```python
from build123d import *

# Parameters (mm, degrees)
ESBO_O1_R                     = 28.25
RESSALTO_EXTRUS_O1_DEPTH      = 12.625
ESBO_O2_R                     = 18.5
CORTE_EXTRUS_O1_DEPTH         = 3.5
ESBO_O3_R                     = 25.75
CORTE_EXTRUS_O2_DEPTH         = 21.75
RESSALTO_EXTRUS_O2_DEPTH      = 9.125
RESSALTO_EXTRUS_O2_DEPTH_BACK = 7.625
ESBO_O4_R                     = 4
FILETE1_R                     = 2.5


with BuildPart() as part:
    # Esboço1 → Ressalto-extrusão1 (new, symmetric)
    with BuildSketch(Plane(origin=(0, 0, 0), x_dir=(1, 0, 0), z_dir=(0, 1, 0))):
        with Locations(Location((0, 0, 0), (0, 0, 270))):
            Circle(ESBO_O1_R)
    extrude(amount=RESSALTO_EXTRUS_O1_DEPTH, both=True)

    # Esboço2 → Corte-extrusão1 (cut)
    with BuildSketch(Plane(origin=(0, 12.625, 0), x_dir=(1, 0, 0), z_dir=(0, 1, 0))):
        with Locations(Location((0, 0, 0), (0, 0, 270))):
            Circle(ESBO_O2_R)
    extrude(amount=-CORTE_EXTRUS_O1_DEPTH, mode=Mode.SUBTRACT)

    # Esboço3 → Corte-extrusão2 (cut)
    with BuildSketch(Plane.XZ.offset(12.625)):
        with Locations(Location((0, 0, 0), (0, 0, 270))):
            Circle(ESBO_O3_R)
    extrude(amount=-CORTE_EXTRUS_O2_DEPTH, mode=Mode.SUBTRACT)

    # Esboço4 → Ressalto-extrusão2 (add, two sides: drawn at the far end of the back side and taken through both)
    with BuildSketch(Plane(origin=(0, 0, 0), x_dir=(1, 0, 0), z_dir=(0, 1, 0)).offset(-RESSALTO_EXTRUS_O2_DEPTH_BACK)):
        with BuildLine():
            Line((4.683419803, 6.111921052), (13.741025404, 21.800154147))
            ThreePointArc((13.741025404, 21.800154147), (12.88470508, 22.316963839), (12.008974596, 22.800154147))
            Line((12.008974596, 22.800154147), (2.951368996, 7.111921052))
            ThreePointArc((2.951368996, 7.111921052), (1.992906647, 7.437628862), (1, 7.634788799))
            Line((1, 7.634788799), (1, 25.75))
            ThreePointArc((1, 25.75), (0, 25.76941016), (-1, 25.75))
            Line((-1, 25.75), (-1, 7.634788799))
            ThreePointArc((-1, 7.634788799), (-1.992906647, 7.437628862), (-2.951368996, 7.111921052))
            Line((-2.951368996, 7.111921052), (-12.008974596, 22.800154147))
            ThreePointArc((-12.008974596, 22.800154147), (-12.88470508, 22.316963839), (-13.741025404, 21.800154147))
            Line((-13.741025404, 21.800154147), (-4.683419803, 6.111921052))
            ThreePointArc((-4.683419803, 6.111921052), (-5.444722215, 5.444722215), (-6.111921052, 4.683419803))
            Line((-6.111921052, 4.683419803), (-21.800154147, 13.741025404))
            ThreePointArc((-21.800154147, 13.741025404), (-22.316963839, 12.88470508), (-22.800154147, 12.008974596))
            Line((-22.800154147, 12.008974596), (-7.111921052, 2.951368996))
            ThreePointArc((-7.111921052, 2.951368996), (-7.437628862, 1.992906647), (-7.634788799, 1))
            Line((-7.634788799, 1), (-25.75, 1))
            ThreePointArc((-25.75, 1), (-25.76941016, 0), (-25.75, -1))
            Line((-25.75, -1), (-7.634788799, -1))
            ThreePointArc((-7.634788799, -1), (-7.437628862, -1.992906647), (-7.111921052, -2.951368996))
            Line((-7.111921052, -2.951368996), (-22.800154147, -12.008974596))
            ThreePointArc((-22.800154147, -12.008974596), (-22.316963839, -12.88470508), (-21.800154147, -13.741025404))
            Line((-21.800154147, -13.741025404), (-6.111921052, -4.683419803))
            ThreePointArc((-6.111921052, -4.683419803), (-5.444722215, -5.444722215), (-4.683419803, -6.111921052))
            Line((-4.683419803, -6.111921052), (-13.741025404, -21.800154147))
            ThreePointArc((-13.741025404, -21.800154147), (-12.88470508, -22.316963839), (-12.008974596, -22.800154147))
            Line((-12.008974596, -22.800154147), (-2.951368996, -7.111921052))
            ThreePointArc((-2.951368996, -7.111921052), (-1.992906647, -7.437628862), (-1, -7.634788799))
            Line((-1, -7.634788799), (-1, -25.75))
            ThreePointArc((-1, -25.75), (0, -25.76941016), (1, -25.75))
            Line((1, -25.75), (1, -7.634788799))
            ThreePointArc((1, -7.634788799), (1.992906647, -7.437628862), (2.951368996, -7.111921052))
            Line((2.951368996, -7.111921052), (12.008974596, -22.800154147))
            ThreePointArc((12.008974596, -22.800154147), (12.88470508, -22.316963839), (13.741025404, -21.800154147))
            Line((13.741025404, -21.800154147), (4.683419803, -6.111921052))
            ThreePointArc((4.683419803, -6.111921052), (5.444722215, -5.444722215), (6.111921052, -4.683419803))
            Line((6.111921052, -4.683419803), (21.800154147, -13.741025404))
            ThreePointArc((21.800154147, -13.741025404), (22.316963839, -12.88470508), (22.800154147, -12.008974596))
            Line((22.800154147, -12.008974596), (7.111921052, -2.951368996))
            ThreePointArc((7.111921052, -2.951368996), (7.437628862, -1.992906647), (7.634788799, -1))
            Line((7.634788799, -1), (25.75, -1))
            ThreePointArc((25.75, -1), (25.76941016, 0), (25.75, 1))
            Line((25.75, 1), (7.634788799, 1))
            ThreePointArc((7.634788799, 1), (7.437628862, 1.992906647), (7.111921052, 2.951368996))
            Line((7.111921052, 2.951368996), (22.800154147, 12.008974596))
            ThreePointArc((22.800154147, 12.008974596), (22.316963839, 12.88470508), (21.800154147, 13.741025404))
            Line((21.800154147, 13.741025404), (6.111921052, 4.683419803))
            ThreePointArc((6.111921052, 4.683419803), (5.444722215, 5.444722215), (4.683419803, 6.111921052))
        make_face()
        with Locations(Location((0, 0, 0), (0, 0, 270))):
            Circle(ESBO_O4_R, mode=Mode.SUBTRACT)
    extrude(amount=RESSALTO_EXTRUS_O2_DEPTH + RESSALTO_EXTRUS_O2_DEPTH_BACK)

    # Filete1
    filete1_edges = [part.edges().sort_by_distance(p)[0] for p in [
        (0, 12.625, -28.25),
    ]]
    fillet(filete1_edges, radius=FILETE1_R)


solid = part.part
```
For this review, take the finished solid that the model builds, in its own axes (mm). A direction names the side the tool comes from. Round coordinates to 2 decimals unless told otherwise and drop trailing zeros. Loops run counter-clockwise (first coordinate to the right, second up) from the corner with the lowest first, then second, coordinate; pieces in that order, holes last.
(1) Tool access review of faces 3 (the cylindrical face through (-7.086, 10.9, 17.089)), 4 (the cylindrical face through (1.98, 0.63, 7.44)), 5 (the flat face through (-21, 9.125, -5)): name each direction out of +Z, -Z, +X, -X, +Y, -Y from which nothing blocks a thin tool from reaching the whole face with its end or side.
Returned:
face 3: +Y
face 4: +Y, -Y
face 5: -Y
(2) Wall thickness on line 1 along Z through (x, y) = (12.5, 7.25); line 2 along X through (y, z) = (-1.5, -13); line 3 along X through (y, z) = (-1.75, 0): over which ranges is each line inside the solid? List them lowest first.
Returned:
line 1: z = -25.33 to -19.65, -8.37 to -6.06, -1 to 1, 6.06 to 8.37, 19.65 to 25.33
line 2: x = -25.08 to -20.52, -8.66 to -6.35, -1 to 1, 6.35 to 8.66, 20.52 to 25.08
line 3: x = -28.25 to -4, 4 to 28.25
(3) Mouldability with a two-part tool opening along Z and no side actions: class faces 1 (the flat face through (-12, -12.625, 23)), 2 (the flat face through (9.144, 0.633, -13.838)) as released by +Z, released by -Z, zero draft, split by the parting line, or undercut.
Returned:
face 1: zero draft
face 2: undercut
(4) We need section A-A (x = 0). Give the boundary of the cut face in (y, z) (3 decimals), plus the area to 3 significant figures.
Returned:
outline: (-12.625, -28.25) - (10.125, -28.25) arc R2.5 ccw to (12.625, -25.75) - (12.625, -18.5) - (9.125, -18.5) - (9.125, -4) - (-7.625, -4) - (-7.625, -25.75) - (-12.625, -25.75) - close; (-12.625, 25.75) - (-7.625, 25.75) - (-7.625, 4) - (9.125, 4) - (9.125, 18.5) - (12.625, 18.5) - (12.625, 25.75) arc R2.5 ccw to (10.125, 28.25) - (-12.625, 28.25) - close
area: 903 mm2
(5) We need section B-B (z = 0). Give the boundary of the cut face in (x, y) (3 decimals).
Returned:
outline: (-28.25, -12.625) - (-25.75, -12.625) - (-25.75, -7.625) - (-4, -7.625) - (-4, 9.125) - (-18.5, 9.125) - (-18.5, 12.625) - (-25.75, 12.625) arc R2.5 ccw to (-28.25, 10.125) - close; (4, -7.625) - (25.75, -7.625) - (25.75, -12.625) - (28.25, -12.625) - (28.25, 10.125) arc R2.5 ccw to (25.75, 12.625) - (18.5, 12.625) - (18.5, 9.125) - (4, 9.125) - close
(6) We need section C-C (y = -8.5). Give the boundary of the cut face in (x, z).
Returned:
outline: circle Ø56.5 at (0, 0); hole circle Ø51.5 at (0, 0)
(7) Clearance check with flat-ended pins moving along their axes: P1, Ø6, axis at x = -13.5, z = 16.5, coming from the -Y side (3 decimals); P2, Ø4.5, axis at x = 4, z = -21, coming from the -Y side (3 decimals); P3, Ø8.5, axis at y = 1.5, z = 15, coming from the +X side; P4, Ø1, axis at x = 14.5, z = 6, coming from the -Y side. State where each tip first meets the part, or that it passes through.
Returned:
P1: stops at y = -7.625
P2: stops at y = 9.125
P3: stops at x = 26.12
P4: passes through
(8) We need section D-D (y = 5). State how many separate pieces and enclosed holes the cut face has, plus the area to 3 significant figures.
Returned:
separate pieces: 1
enclosed holes: 13
area: 994 mm2
